Geometry check sheet. Reference: the model listing, model coordinates, mm. Face numbers are marked on the shaded views. A direction names the side the tool comes from. Coordinates: 2 decimals unless noted, no trailing zeros. Order: outer loops, then holes, each group sorted by start corner. A loop starts at its lowest first (then second) coordinate and runs counter-clockwise, first axis right, second up. Notation, with made-up numbers: M 3,-12 L 59,-12 A24 cw 59,3 Z; hole C -34.75,21 d9. An arc over 180 degrees is marked long. One line per item, written item: value. Start each with the question number.
1) Sectioned sample at C-C, the plane y = 0. Enter the section's corners in (x, z) (1 decimal).
2) Go/stop test with flat-tipped pins: P1, Ø7.5, axis at x = -14, y = 0.5, coming from the +Z side; P2, Ø5.5, axis at x = 15.875, y = 0, coming from the +Z side. Record where each tip stops, or that it passes through.
3) Thickness scan on L1, parallel to Y at x = -15.5, z = 3.5; L2, parallel to X at y = -6, z = 4.1 (3 decimals); L3, parallel to Y at x = -18.5, z = 3.2. Record the ranges inside material, lowest first. Write a range as from..to.
4) Sectioned sample at A-A, the plane z = 1.1. State how many separate pieces and enclosed holes the cut face has, then the cut area to 3 significant figures.
5) Draft check along Y on the marked faces 3 and 4. Enter one of: pulls with the +Y half, pulls with the -Y half, needs draft (parallel to the pull), parting line crosses it, or undercut.
6) Access from +Z, -Z, +X, -X, +Y, -Y to the whole of each face (thin tool, end or side, straight path). Record for the marked faces 1 and 2.
7) Sectioned sample at D-D, the plane x = 16. Enter the section's corners in (y, z).
```python
from build123d import *

# Parameters (mm, degrees)
SKETCH1_W           = 69.85
SKETCH1_H           = 63.5
SKETCH1_R           = 2.4892
BOSS_EXTRUDE1_DEPTH = 4.7625
CHAMFER1_SIZE       = 3.175
SKETCH2_R           = 4.7625
CUT_EXTRUDE1_DEPTH  = 2.38125


with BuildPart() as part:
    # Sketch1 → Boss-Extrude1 (new body)
    with BuildSketch(Plane.XY):
        Rectangle(SKETCH1_W, SKETCH1_H)
        with Locations(Location((-15.875, 0, 0), (0, 0, 180))):
            Circle(SKETCH1_R, mode=Mode.SUBTRACT)
        with Locations(Location((15.875, 0, 0), (0, 0, 180))):
            Circle(SKETCH1_R, mode=Mode.SUBTRACT)
        with BuildLine():
            Line((7.9375, 1.5875), (7.9375, -1.5875))
            ThreePointArc((7.9375, -1.5875), (0, -9.525), (-7.9375, -1.5875))
            Line((-7.9375, -1.5875), (-7.9375, 1.5875))
            ThreePointArc((-7.9375, 1.5875), (0, 9.525), (7.9375, 1.5875))
        make_face(mode=Mode.SUBTRACT)
    extrude(amount=BOSS_EXTRUDE1_DEPTH)

    # Chamfer1
    chamfer1_edges = [part.edges().sort_by_distance(p)[0] for p in [
        (34.925, -31.75, 2.38125),
        (-34.925, -31.75, 2.38125),
        (-34.925, 31.75, 2.38125),
        (34.925, 31.75, 2.38125),
    ]]
    chamfer(chamfer1_edges, length=CHAMFER1_SIZE)

    # Sketch2 → Cut-Extrude1 (cut)
    with BuildSketch(Plane.XY.offset(4.7625)):
        with Locations((-15.875, 0)):
            Circle(SKETCH2_R)
        with Locations((15.875, 0)):
            Circle(SKETCH2_R)
    extrude(amount=-CUT_EXTRUDE1_DEPTH, mode=Mode.SUBTRACT)


solid = part.part
```
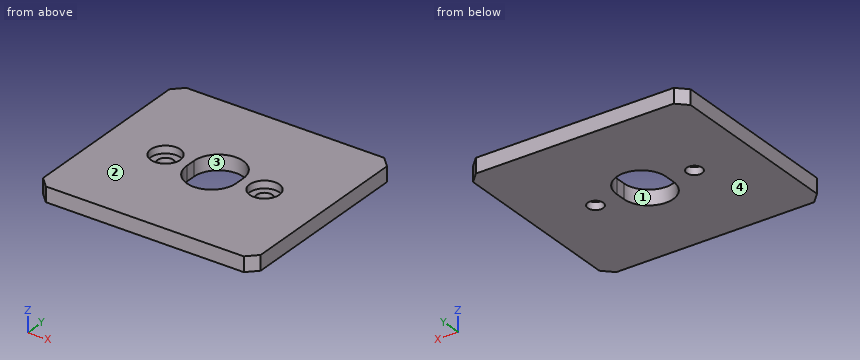
Final values:
1. outline: M -34.9,0 L -18.4,0 L -18.4,2.4 L -20.6,2.4 L -20.6,4.8 L -34.9,4.8 Z; M -13.4,0 L -7.9,0 L -7.9,4.8 L -11.1,4.8 L -11.1,2.4 L -13.4,2.4 Z; M 7.9,0 L 13.4,0 L 13.4,2.4 L 11.1,2.4 L 11.1,4.8 L 7.9,4.8 Z; M 18.4,0 L 34.9,0 L 34.9,4.8 L 20.6,4.8 L 20.6,2.4 L 18.4,2.4 Z
2. P1: stops at z = 4.76
2. P2: stops at z = 2.38
3. L1: y = -31.75..-4.75, 4.75..31.75
3. L2: x = -34.925..-6.598, 6.598..34.925
3. L3: y = -31.75..-3.97, 3.97..31.75
4. separate pieces: 1
4. enclosed holes: 3
4. area: 4,130 mm^2
5. face 3: undercut
5. face 4: needs draft
6. face 1: +Z, -Z
6. face 2: +Z, +X, -X, +Y, -Y
7. outline: M -31.75,0 L -2.49,0 L -2.49,2.38 L -4.76,2.38 L -4.76,4.76 L -31.75,4.76 Z; M 2.49,0 L 31.75,0 L 31.75,4.76 L 4.76,4.76 L 4.76,2.38 L 2.49,2.38 Z
